Source: CAD feature listing. Evaluate the final solid. Frame: model axes, mm. Coordinates: 2 decimals unless noted, no trailing zeros. Write each loop counter-clockwise with the first axis right and the second up, starting at its lowest first coordinate (ties: lowest second). Pieces come first, ordered by that corner, then holes. Notation, with made-up numbers: (38.25, 40) -> (48.25, 40) arc R12 cw to (48.25, 60) -> close; hole circle Ø7 at (37, 31.5). An arc over 180 degrees is marked (long way). One line per item, written item: value. Start each with the question number.
1. First-contact query: P1, Ø1.8, axis at x = -44.1, z = -48.05, coming from the +Y side. Flat tip, straight axial feed; report the tip coordinate or a pass-through.
2. Mould query, pull axis X, two halves, no side actions, for faces 1 (the flat face through (-1, 1, -53.05)), 2 (the flat face through (74.1, 1, 1)), 3 (the cylindrical face through (-45.01, 1.48, 49.24)). Classes: released by +X, released by -X, zero draft, split by the parting line, or undercut.
3. Section query A-A, the plane x = 32.3. Output: boundary loops of the cut face in (y, z).
4. Section query B-B, the plane z = 48.05. Output: boundary loops of the cut face in (x, y), and give its area (3 significant figures).
5. Line query: line 1 (X direction, y = 1.2, z = 48.05). Output: solid intervals per line, ascending.
6. Section query C-C, the plane x = -69.1. Output: boundary loops of the cut face in (y, z).
from build123d import *

# Parameters (mm, degrees)
SKETCH1_W           = 148.2
SKETCH1_H           = 106.1
SKETCH1_R           = 1.6
BOSS_EXTRUDE1_DEPTH = 3
FILLET1_R           = 2
CUT_EXTRUDE1_REACH  = 93.182
SKETCH3_R           = 1.5


with BuildPart() as part:
    # Sketch1 → Boss-Extrude1 (new body)
    with BuildSketch(Plane(origin=(0, 0, 0), x_dir=(1, 0, 0), z_dir=(0, 1, 0))):
        Rectangle(SKETCH1_W, SKETCH1_H)
        with Locations(Location((-69.1, 48.05, 0), (0, 0, 270))):
            Circle(SKETCH1_R, mode=Mode.SUBTRACT)
        with Locations(Location((-69.1, -48.05, 0), (0, 0, 90))):
            Circle(SKETCH1_R, mode=Mode.SUBTRACT)
        with Locations(Location((69.1, -48.05, 0), (0, 0, 270))):
            Circle(SKETCH1_R, mode=Mode.SUBTRACT)
        with Locations(Location((69.1, 48.05, 0), (0, 0, 90))):
            Circle(SKETCH1_R, mode=Mode.SUBTRACT)
    extrude(amount=BOSS_EXTRUDE1_DEPTH)

    # Fillet1
    fillet1_edges = [part.edges().sort_by_distance(p)[0] for p in [
        (-74.1, 1.5, -53.05),
        (74.1, 1.5, -53.05),
        (74.1, 1.5, 53.05),
        (-74.1, 1.5, 53.05),
    ]]
    fillet(fillet1_edges, radius=FILLET1_R)

    # Sketch3 → Cut-Extrude1 (cut, up to next)
    with BuildSketch(Plane.XZ, mode=Mode.PRIVATE) as cut_extrude1_sk1:
        with Locations(Location((32.3, 48.05, 0), (0, 0, 270))):
            Circle(SKETCH3_R)
    cut_extrude1_tool1 = extrude(cut_extrude1_sk1.sketch, amount=-CUT_EXTRUDE1_REACH, mode=Mode.PRIVATE) & part.part
    # Sketch3 → Cut-Extrude1 (cut, up to next)
    with BuildSketch(Plane.XZ, mode=Mode.PRIVATE) as cut_extrude1_sk2:
        with Locations(Location((-44.1, 48.05, 0), (0, 0, 270))):
            Circle(SKETCH3_R)
    cut_extrude1_tool2 = extrude(cut_extrude1_sk2.sketch, amount=-CUT_EXTRUDE1_REACH, mode=Mode.PRIVATE) & part.part
    # Sketch3 → Cut-Extrude1 (cut, up to next)
    with BuildSketch(Plane.XZ, mode=Mode.PRIVATE) as cut_extrude1_sk3:
        with Locations(Location((-44.1, -48.05, 0), (0, 0, 270))):
            Circle(SKETCH3_R)
    cut_extrude1_tool3 = extrude(cut_extrude1_sk3.sketch, amount=-CUT_EXTRUDE1_REACH, mode=Mode.PRIVATE) & part.part
    # Sketch3 → Cut-Extrude1 (cut, up to next)
    with BuildSketch(Plane.XZ, mode=Mode.PRIVATE) as cut_extrude1_sk4:
        with Locations(Location((32.3, -48.05, 0), (0, 0, 270))):
            Circle(SKETCH3_R)
    cut_extrude1_tool4 = extrude(cut_extrude1_sk4.sketch, amount=-CUT_EXTRUDE1_REACH, mode=Mode.PRIVATE) & part.part
    add(cut_extrude1_tool1.solids().sort_by_distance((32.3, 0, 48.05))[0], mode=Mode.SUBTRACT)
    add(cut_extrude1_tool2.solids().sort_by_distance((-44.1, 0, 48.05))[0], mode=Mode.SUBTRACT)
    add(cut_extrude1_tool3.solids().sort_by_distance((-44.1, 0, -48.05))[0], mode=Mode.SUBTRACT)
    add(cut_extrude1_tool4.solids().sort_by_distance((32.3, 0, -48.05))[0], mode=Mode.SUBTRACT)


solid = part.part
Computed values:
1. P1: passes through
2. face 1: zero draft
2. face 2: released by +X
2. face 3: undercut
3. outline: (0, -53.05) -> (3, -53.05) -> (3, -49.55) -> (0, -49.55) -> close; (0, -46.55) -> (3, -46.55) -> (3, 46.55) -> (0, 46.55) -> close; (0, 49.55) -> (3, 49.55) -> (3, 53.05) -> (0, 53.05) -> close
4. outline: (-74.1, 0) -> (-70.7, 0) -> (-70.7, 3) -> (-74.1, 3) -> close; (-67.5, 0) -> (-45.6, 0) -> (-45.6, 3) -> (-67.5, 3) -> close; (-42.6, 0) -> (30.8, 0) -> (30.8, 3) -> (-42.6, 3) -> close; (33.8, 0) -> (67.5, 0) -> (67.5, 3) -> (33.8, 3) -> close; (70.7, 0) -> (74.1, 0) -> (74.1, 3) -> (70.7, 3) -> close
4. area: 407 mm²
5. line 1: x = -74.1 to -70.7, -67.5 to -45.6, -42.6 to 30.8, 33.8 to 67.5, 70.7 to 74.1
6. outline: (0, -53.05) -> (3, -53.05) -> (3, -49.65) -> (0, -49.65) -> close; (0, -46.45) -> (3, -46.45) -> (3, 46.45) -> (0, 46.45) -> close; (0, 49.65) -> (3, 49.65) -> (3, 53.05) -> (0, 53.05) -> close
